For this review, take the finished solid that the model builds, in its own axes (mm). Face numbers are marked on the shaded views. A direction names the side the tool comes from. Give positions to 0.01 mm unless a question says otherwise; leave off trailing zeros. Write each loop counter-clockwise with the first axis right and the second up, starting at its lowest first coordinate (ties: lowest second). Pieces come first, ordered by that corner, then holes.
1) We need section C-C on y = 7.5. Give the boundary of the cut face in (x, z), and give its area (3 significant figures).
2) We need section A-A on x = 41.25. Give the boundary of the cut face in (y, z).
3) Draft analysis for pull direction Y (two halves, no side actions). For the marked faces 1, 2, 3 and 4, state which applies: pulls with the +Y half, pulls with the -Y half, needs draft (parallel to the pull), parting line crosses it, or undercut.
4) We need section D-D on y = 16. Give the boundary of the cut face in (x, z), and give its area (3 significant figures).
5) For P1, Ø4, axis at x = 56.5, z = 17.5, coming from the -Y side; P2, Ø10, axis at x = 41.25, y = 27.5, coming from the -Z side; P3, Ø2, axis at y = 27, z = 4, coming from the -X side; P4, Ø3.5, axis at x = 18.5, y = 25, coming from the +Z side, all flat-tipped, find the tip position at first contact; note any pin that passes through.
6) We need section B-B on z = 33. Give the boundary of the cut face in (x, y), and give its area (3 significant figures).
7) Wall thickness on line 1 along Y through (x, z) = (30, 1.75); line 2 along X through (y, z) = (27.5, 0.1); line 3 along X through (y, z) = (36, 28.5): over which ranges is each line inside the solid? List them lowest first.
8) Machinability: for the marked faces 5, 6, 7, 8 and 9, which of the approach directions +Z, -Z, +X, -X, +Y, -Y give a long, thin tool a straight path to every point of the face, cutting with its end or side? Answer none if there is none.
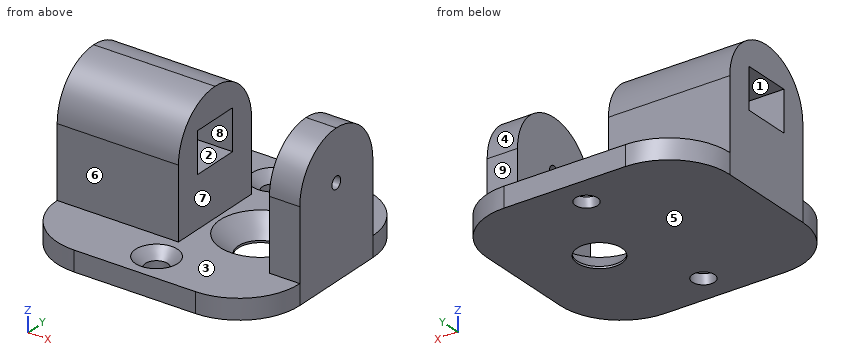
Autodesk Fusion 360 part; units mm, degrees
sketch "Skizze3" plane through (0, 0, 0) normal (0, 0, 1) x (1, 0, 0)
  line L0 (0, 0) -> (60, 0)
  line L1 (60, 0) -> (60, 55)
  line L2 (60, 55) -> (0, 55)
  line L3 (0, 55) -> (0, 0)
  line L4 (60, 55) -> (0, 55)
  line L5 (0, 55) -> (0, 0)
  line L6 (0, 0) -> (60, 0)
  line L7 (60, 0) -> (60, 55)
  line L8 (0, 15) -> (60, 15)
  line L9 (0, 40) -> (60, 40)
  line L10 (30, 40) -> (52.5, 40)
  line L11 (52.5, 40) -> (52.5, 15)
  line L12 (52.5, 15) -> (30, 15)
  line L13 (30, 15) -> (30, 40)
  point P0 (30, 7.5)
  point P1 (30, 47.5)
  dimension "d5" = 55
  dimension "d6" = 60
  dimension "d11" = 7.5
  dimension "d12" = 7.5
  dimension "d13" = 30
  dimension "d14" = 30
  dimension "d15" = 15
  dimension "d16" = 15
  dimension "d17" = 30
  dimension "d18" = 7.5
  dimension "d19" = 22.5
extrude "Extrusion2" add sketch "Skizze3" along normal blind 5
fillet "Abrundung2" radius 15 4 edges at (0, 55, 2.5) (0, 0, 2.5) (60, 0, 2.5) (60, 55, 2.5)
sketch "Skizze4" plane through (0, 0, 0) normal (0, 0, 1) x (1, 0, 0)
  line L0 (0, 15) -> (30, 15)
  line L1 (30, 15) -> (30, 40)
  line L2 (30, 40) -> (0, 40)
  line L3 (0, 40) -> (0, 15)
  point P0 (0, 15)
  point P1 (30, 40)
sketch "Skizze5" plane through (0, 0, 5) normal (0, 0, 1) x (-1, 0, 0)
  arc A0 (-60, -40) -> (-45, -55) centre (-45, -40) ccw
  line L0 (-45, -55) -> (-15, -55)
  arc A1 (-15, -55) -> (0, -40) centre (-15, -40) ccw
  line L1 (0, -40) -> (0, -15)
  arc A2 (0, -15) -> (-15, 0) centre (-15, -15) ccw
  line L2 (-15, 0) -> (-45, 0)
  arc A3 (-45, 0) -> (-60, -15) centre (-45, -15) ccw
  line L3 (-60, -15) -> (-60, -40)
  line L4 (-60, -15) -> (-52.5, -15)
  line L5 (-52.5, -15) -> (-52.5, -40)
  line L6 (-52.5, -40) -> (-60, -40)
  line L7 (-60, -40) -> (-60, -15)
  dimension "d20" = 7.5
  dimension "d21" = 25
extrude "Extrusion3" add sketch "Skizze5" along normal blind 30 contours L3 L4 L5 L6 L7
fillet "Abrundung3" radius 12.5 2 edges at (56.25, 15, 35) (56.25, 40, 35)
extrude "Extrusion4" add sketch "Skizze3" along normal blind 35 contours L3 L5 L8 L9 L13
fillet "Abrundung4" radius 12.5 2 edges at (15, 15, 35) (15, 40, 35)
sketch "Skizze6" plane through (0, 0, 5) normal (0, 0, 1) x (-1, 0, 0)
  line L0 (-30, -15) -> (0, -15)
  arc A0 (0, -15) -> (-15, 0) centre (-15, -15) ccw
  line L1 (-15, 0) -> (-45, 0)
  arc A1 (-45, 0) -> (-60, -15) centre (-45, -15) ccw
  line L2 (-60, -15) -> (-52.5, -15)
  line L3 (-52.5, -15) -> (-52.5, -40)
  line L4 (-52.5, -40) -> (-60, -40)
  arc A2 (-60, -40) -> (-45, -55) centre (-45, -40) ccw
  line L5 (-45, -55) -> (-15, -55)
  arc A3 (-15, -55) -> (0, -40) centre (-15, -40) ccw
  line L6 (0, -40) -> (-30, -40)
  line L7 (-30, -40) -> (-30, -15)
  point P0 (-30, -7.5)
  point P1 (-30, -47.5)
  point P2 (-41.25, -27.5)
  dimension "d48" = 27.5
  dimension "d49" = 27.5
  dimension "d50" = 11.25
  dimension "d51" = 11.25
hole "Bohrung1" at (30, 7.5, 5) at (30, 47.5, 5) direction (0, 0, -1) diameter 5.5 depth 33 tip angle 180 countersink diameter 10.4 countersink angle 90
sketch "Skizze7" plane through (60, 0, 0) normal (1, 0, 0) x (0, 1, 0)
  arc A0 (40, 22.5) -> (27.5, 35) centre (27.5, 22.5) ccw
  arc A1 (27.5, 35) -> (15, 22.5) centre (27.5, 22.5) ccw
  line L0 (15, 22.5) -> (15, 5)
  line L1 (15, 5) -> (15, 0)
  line L2 (15, 0) -> (40, 0)
  line L3 (40, 0) -> (40, 5)
  line L4 (40, 5) -> (40, 22.5)
  line L5 (0, 0) -> (55, 0)
  point P0 (27.5, 22.5)
  dimension "d35" = 12.5
  dimension "d36" = 22.5
hole "Bohrung2" at (60, 27.5, 22.5) direction (-1, 0, 0) diameter 3 depth 33 tip angle 180
sketch "Skizze8" plane through (0, 0, 0) normal (-1, 0, 0) x (0, -1, 0)
  arc A0 (-27.5, 35) -> (-40, 22.5) centre (-27.5, 22.5) ccw
  line L0 (-40, 22.5) -> (-40, 5)
  line L1 (-40, 5) -> (-40, 0)
  line L2 (-40, 0) -> (-15, 0)
  line L3 (-15, 0) -> (-15, 5)
  line L4 (-15, 5) -> (-15, 22.5)
  arc A1 (-15, 22.5) -> (-27.5, 35) centre (-27.5, 22.5) ccw
  line L5 (-33.5, 27.5) -> (-21.5, 27.5)
  line L6 (-21.5, 27.5) -> (-21.5, 17.5)
  line L7 (-21.5, 17.5) -> (-33.5, 17.5)
  line L8 (-33.5, 17.5) -> (-33.5, 27.5)
  line L9 (-55, 0) -> (0, 0)
  dimension "d40" = 12
  dimension "d41" = 10
  dimension "d42" = 6.5
  dimension "d43" = 6.5
  dimension "d44" = 17.5
  dimension "d45" = 7.5
extrude "Extrusion5" cut sketch "Skizze8" against normal blind 30 contours L5 L6 L7 L8
sketch "Skizze9" plane through (0, 0, 0) normal (0, 0, 1) x (1, 0, 0)
  point P0 (42.3928, 28.246)
  point P1 (43.9941, 27.6171)
hole "Bohrung3" at (41.25, 27.5, 5) direction (0, 0, -1) diameter 11 depth 10 tip angle 180 countersink diameter 20 countersink angle 90
extrude "Extrusion1" [suppressed]
fillet "Abrundung1" [suppressed]
Results list:
1. outline: (2.01, 0) - (27.25, 0) - (27.25, 2.55) - (24.8, 5) - (2.01, 5) - close; (32.75, 0) - (57.99, 0) - (57.99, 5) - (35.2, 5) - (32.75, 2.55) - close
1. area: 246 mm2
2. outline: (0, 0) - (22, 0) - (22, 0.5) - (17.5, 5) - (0, 5) - close; (33, 0) - (55, 0) - (55, 5) - (37.5, 5) - (33, 0.5) - close
3. face 1: undercut
3. face 2: undercut
3. face 3: needs draft
3. face 4: pulls with the +Y half
4. outline: (0, 0) - (60, 0) - (60, 27.4) - (52.5, 27.4) - (52.5, 5) - (30, 5) - (30, 27.4) - (0, 27.4) - close
4. area: 1,140 mm2
5. P1: stops at y = 15
5. P2: passes through
5. P3: stops at x = 0
5. P4: stops at z = 34.98
6. outline: (0, 20.72) - (30, 20.72) - (30, 34.28) - (0, 34.28) - close; (52.5, 20.72) - (60, 20.72) - (60, 34.28) - (52.5, 34.28) - close
6. area: 509 mm2
7. line 1: y = 0 to 4.75, 10.25 to 44.75, 50.25 to 55
7. line 2: x = 0 to 35.75, 46.75 to 60
7. line 3: x = 0 to 30, 52.5 to 60
8. face 5: -Z, +X, -X, +Y, -Y
8. face 6: +Z, +X, -X, -Y
8. face 7: +Z, +Y, -Y
8. face 8: -X
8. face 9: +Z, +X, -X, +Y
